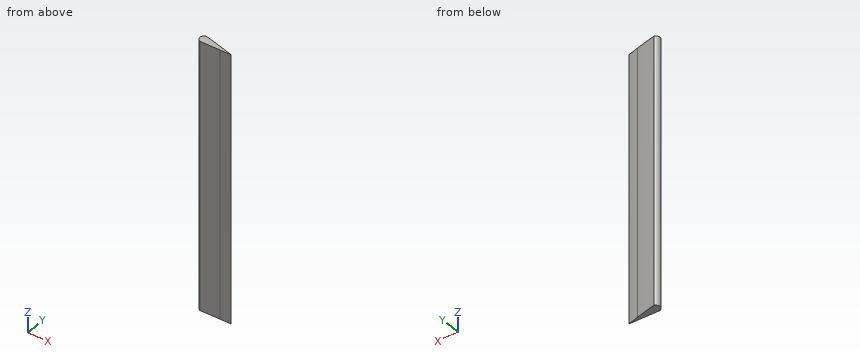
from build123d import *

# Parameters (mm, degrees)
BOSS_EXTRUDE1_DEPTH = 249


with BuildPart() as part:
    # Sketch1 → Boss-Extrude1 (new body)
    with BuildSketch(Plane.XY):
        with BuildLine():
            Line((189.698329187, 23.077647259), (207.849600842, 23.11245238))
            Line((207.849600842, 23.11245238), (217.965296171, 23.11245238))
            Line((217.965296171, 23.11245238), (208.199662873, 25.963149641))
            add(Edge.make_bspline(
                [(208.199662873, 25.963149641), (205.461210323, 26.762534479), (203.172469982, 27.404419223), (200.508776125, 28.151460912), (198.127071623, 28.777602141), (193.949594484, 29.875845298), (189.698329187, 30.854494337)],
                knots=[0, 0, 0, 0.25, 0.25, 0.5, 0.5, 0.915466563, 0.915466563, 0.915466563], degree=2))
            ThreePointArc((189.698329187, 30.854494337), (186.628644326, 26.966070798), (189.698329187, 23.077647259))
        make_face()
    extrude(amount=BOSS_EXTRUDE1_DEPTH)


solid = part.part
CAD build for the part. Positions are in the model's coordinates, mm. Round coordinates to 2 decimals unless told otherwise and drop trailing zeros. Loops run counter-clockwise (first coordinate to the right, second up) from the corner with the lowest first, then second, coordinate; pieces in that order, holes last. Notation, with made-up numbers: M 27.5,3.25 L 59.5,3.25 A27 cw 59.5,31.25 Z; hole C -3.75,60.5 d7. An arc over 180 degrees is marked long. One line per question, with ' | ' between items. Start each with the question number.
Item 1: Pin check, flat tips, straight feed: pin 1 Ø1.5 at (x, z) = (205.5, 30) entering from +Y; pin 2 Ø3 at (x, z) = (215, 105.5) entering from -Y. Stop position of each tip, or through.
Item 2: Cut at A-A, the plane x = 212. Write the cut outline in (y, z).
Item 3: Wall check: line 1 (Y direction, x = 212, z = 21.5); line 2 (Y direction, x = 197.5, z = 48). Give the ranges that are in metal, low to high.
Responses:
1) pin 1: stops at y = 26.96 | pin 2: stops at y = 23.11
2) outline: M 23.11,0 L 24.85,0 L 24.85,249 L 23.11,249 Z
3) line 1: y = 23.11 to 24.85 | line 2: y = 23.09 to 28.94
